Source: three-view drawing plus pictorial views. Frame: mm from the lowest corner of the part. A direction names the side the tool comes from. Give positions to 0.01 mm unless a question says otherwise; leave off trailing zeros. Loops run counter-clockwise (first coordinate to the right, second up) from the corner with the lowest first, then second, coordinate; pieces in that order, holes last.
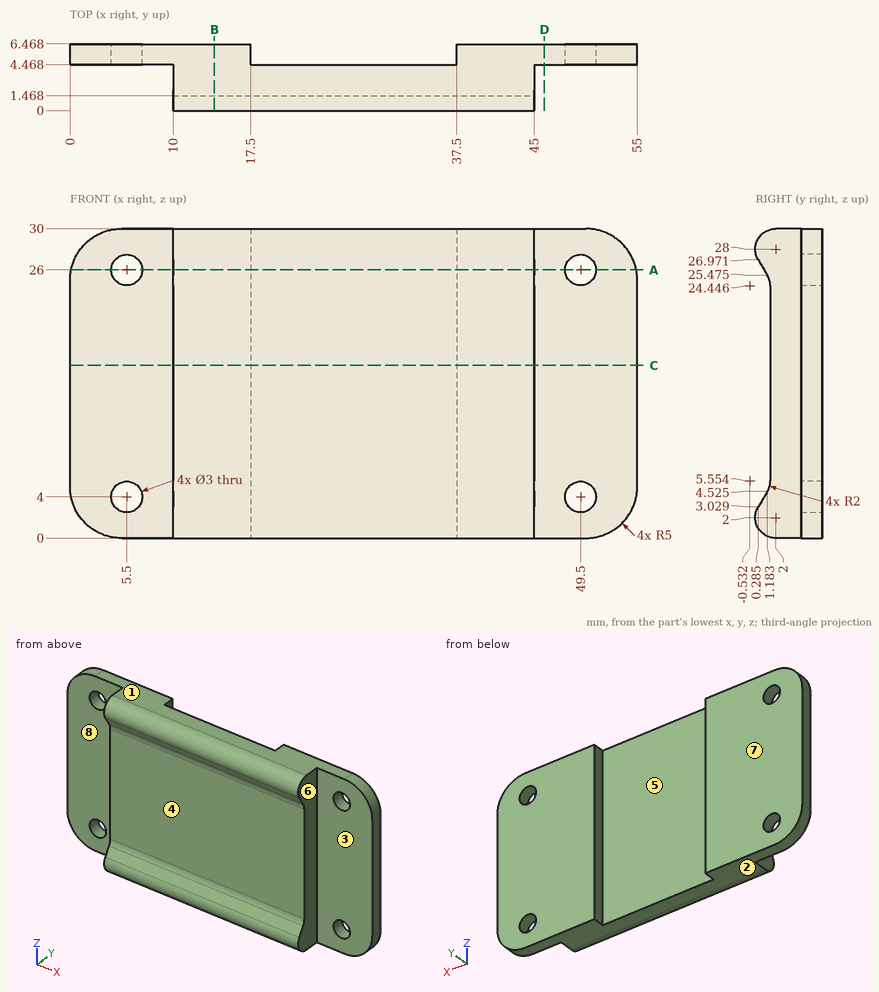
1) Contact query for flat-ended pins moving along their axis: P1, Ø6, axis at x = 23.5, z = 16, coming from the +Y side; P2, Ø3.5, axis at x = 49.5, z = 4, coming from the -Y side; P3, Ø1.5, axis at y = 5, z = 3.5, coming from the +X side; P4, Ø3.5, axis at y = 3, z = 9, coming from the +X side. Output: stop coordinate, or through.
Checks:
P1: stops at y = 4.47
P2: stops at y = 4.47
P3: stops at x = 54.94
P4: stops at x = 55
2) Pull-direction query (Z, two-part tool) for the marked faces 1, 2, 3 and 4; classes: released by +Z, released by -Z, zero draft, split by the parting line, or undercut.
Checks:
face 1: released by +Z
face 2: released by -Z
face 3: zero draft
face 4: undercut
3) Cut plane A-A (z = 26). Return loops of the section in (x, y).
Checks:
outline: (0.1, 4.47) - (4, 4.47) - (4, 6.47) - (0.1, 6.47) - close; (7, 4.47) - (10, 4.47) - (10, 0.87) - (45, 0.87) - (45, 4.47) - (48, 4.47) - (48, 6.47) - (37.5, 6.47) - (37.5, 4.47) - (17.5, 4.47) - (17.5, 6.47) - (7, 6.47) - close; (51, 4.47) - (54.9, 4.47) - (54.9, 6.47) - (51, 6.47) - close
4) Cut plane D-D (x = 46). Return loops of the section in (y, z).
Checks:
outline: (4.47, 0) - (6.47, 0) - (6.47, 30) - (4.47, 30) - close
5) Reachability of the marked faces 5, 6, 7 and 8 from +Z, -Z, +X, -X, +Y, -Y: full face, straight path, thin tool, end or side. Return the list, or none.
Checks:
face 5: +Z, -Z, +Y
face 6: +Z, -Z, +X, -Y
face 7: +Z, -Z, +X, -X, +Y
face 8: +Z, -Z, -X, -Y
6) Ray query, probe 1 along X at (y, z) = (5.5, 13); probe 2 along X at (y, z) = (5.6, 4); probe 3 along Y at (x, z) = (16.5, 23.25). Return the intervals inside material, ascending.
Checks:
probe 1: x = 0 to 17.5, 37.5 to 55
probe 2: x = 0.1 to 4, 7 to 17.5, 37.5 to 48, 51 to 54.9
probe 3: y = 1.47 to 6.47
7) Cut plane B-B (x = 14). Return loops of the section in (y, z) (1 decimal), and give its area (3 significant figures).
Checks:
outline: (0.3, 3) arc R2 ccw to (2, 0) - (6.5, 0) - (6.5, 30) - (2, 30) arc R2 ccw to (0.3, 27) - (1.2, 25.5) arc R2 cw to (1.5, 24.4) - (1.5, 5.6) arc R2 cw to (1.2, 4.5) - close
area: 159 mm2
8) Cut plane C-C (z = 16.75). Return loops of the section in (x, y), and give its area (3 significant figures).
Checks:
outline: (0, 4.47) - (10, 4.47) - (10, 1.47) - (45, 1.47) - (45, 4.47) - (55, 4.47) - (55, 6.47) - (37.5, 6.47) - (37.5, 4.47) - (17.5, 4.47) - (17.5, 6.47) - (0, 6.47) - close
area: 175 mm2
